Answer from the drawing. Dimensions are ordinates in mm from the lowest x, y and z of the part. Coordinates: 2 decimals unless noted, no trailing zeros. Write each loop counter-clockwise with the first axis right and the second up, starting at its lowest first coordinate (ties: lowest second). Pieces come first, ordered by that corner, then holes.
(1) The part is cut by section A-A, the plane x = 3. Determine the outline of the cut face in (y, z), and give its area (4 significant figures).
(2) A straight line is drawn through the part: line 1 along X through (y, z) = (4, 9). Find the intervals that lie inside material, in ascending order.
(3) Given pin 1 (1.5 mm diameter, centred on x = 3, z = 8.5, fed in from -Y), flat-ended and moving along its own axis, determine where the tip first touches the part or whether it passes through.
(4) The part is cut by section B-B, the plane z = 36. Determine the outline of the cut face in (x, y).
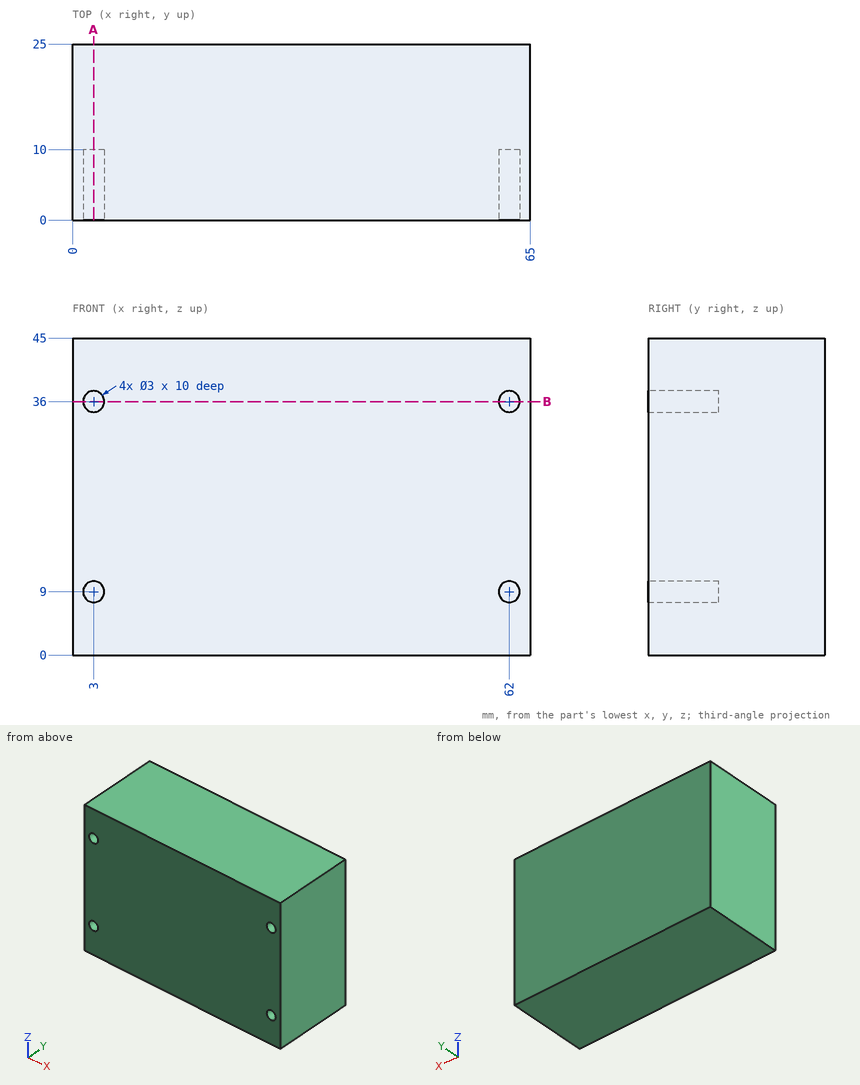
Computed:
1. outline: (0, 0) - (25, 0) - (25, 45) - (0, 45) - (0, 37.5) - (10, 37.5) - (10, 34.5) - (0, 34.5) - (0, 10.5) - (10, 10.5) - (10, 7.5) - (0, 7.5) - close
1. area: 1,065 mm2
2. line 1: x = 0 to 1.5, 4.5 to 60.5, 63.5 to 65
3. pin 1: stops at y = 10
4. outline: (0, 0) - (1.5, 0) - (1.5, 10) - (4.5, 10) - (4.5, 0) - (60.5, 0) - (60.5, 10) - (63.5, 10) - (63.5, 0) - (65, 0) - (65, 25) - (0, 25) - close
